from build123d import *

# Parameters (mm, degrees)
BOSS_EXTRUDE1_DEPTH = 600
FILLET1_R           = 5


with BuildPart() as part:
    # Sketch1 → Boss-Extrude1 (new body)
    with BuildSketch(Plane.XY):
        Polygon((-37.5, 50), (37.5, 50), (37.5, 40), (5, 34.269373127), (5, -34.269373127), (37.5, -40), (37.5, -50), (-37.5, -50), (-37.5, -40), (-5, -34.269373127), (-5, 34.269373127), (-37.5, 40), align=None)
    extrude(amount=BOSS_EXTRUDE1_DEPTH)

    # Fillet1
    fillet1_edges = [part.edges().sort_by_distance(p)[0] for p in [
        (5, 34.269373127, 300),
        (5, -34.269373127, 300),
        (37.5, -40, 300),
        (-37.5, -40, 300),
        (-5, -34.269373127, 300),
        (-5, 34.269373127, 300),
        (-37.5, 40, 300),
        (37.5, 40, 300),
    ]]
    fillet(fillet1_edges, radius=FILLET1_R)


solid = part.part
Input: part model. Units: mm. Frame: model coordinates. A direction names the side the tool comes from. Coordinates: 2 decimals unless noted, no trailing zeros. Order: outer loops, then holes, each group sorted by start corner. A loop starts at its lowest first (then second) coordinate and runs counter-clockwise, first axis right, second up. Notation, with made-up numbers: M 82.25,-5.75 L 138.25,-5.75 A21 ccw 138.25,3.25 Z; hole C 9.25,14.25 d10. An arc over 180 degrees is marked long. Write item = value, one per line. Start each with the question number.
(1) First-contact query: P1, Ø12, axis at y = -15, z = 436, coming from the +X side; P2, Ø2, axis at y = 12, z = 184.5, coming from the -X side; P3, Ø8, axis at x = 14, y = 36, coming from the -Z side. Flat tips, straight axial feed; report the tip coordinate or a pass-through.
(2) Line query: line 1 along X through (y, z) = (-5.5, 460); line 2 along Y through (x, z) = (-7.5, 305.5); line 3 along X through (y, z) = (-43.5, 83). Output: solid intervals per line, ascending. Write a range as [from, to].
(3) Section C-C on y = -8. Output: boundary loops of the cut face in (x, z), and give its area (3 significant figures).
(4) Pull-direction query (Y, two-part tool) for faces 4 (the flat face through (0, -3, 0)), 5 (the flat face through (-21.42, -37.165, 295.8)), 6 (the flat face through (-1, 50, 296)), 7 (the flat face through (-5, 0, 296)); classes: released by +Y, released by -Y, zero draft, split by the parting line, or undercut.
(5) Section B-B on z = 178. Output: boundary loops of the cut face in (x, y).
(6) Reachability of faces 1 (the flat face through (-21.08, 37.105, 295.8)), 2 (the flat face through (21.42, 37.165, 295.8)), 3 (the flat face through (0, -3, 600)) from +Z, -Z, +X, -X, +Y, -Y: full face, straight path, thin tool, end or side. Return the list, or none.
(7) Section A-A on x = -18. Output: boundary loops of the cut face in (y, z).
Result set:
q1.P1 = 5
q1.P2 = -5
q1.P3 = 0
q2.line_1 = [-5, 5]
q2.line_2 = [-50, -34.4], [34.4, 50]
q2.line_3 = [-37.45, 37.45]
q3.outline = M -5,0 L 5,0 L 5,600 L -5,600 Z
q3.area = 6,000 mm²
q4.face_4 = zero draft
q4.face_5 = undercut
q4.face_6 = released by +Y
q4.face_7 = undercut
q5.outline = M -37.5,-50 L 37.5,-50 L 37.5,-44.2 A5 ccw 33.37,-39.27 L 9.13,-35 A5 cw 5,-30.07 L 5,30.07 A5 cw 9.13,35 L 33.37,39.27 A5 ccw 37.5,44.2 L 37.5,50 L -37.5,50 L -37.5,44.2 A5 ccw -33.37,39.27 L -9.13,35 A5 cw -5,30.07 L -5,-30.07 A5 cw -9.13,-35 L -33.37,-39.27 A5 ccw -37.5,-44.2 Z
q6.face_1 = +Z, -Z, -X
q6.face_2 = +Z, -Z, +X
q6.face_3 = +Z, +X, -X, +Y, -Y
q7.outline = M -50,0 L -36.56,0 L -36.56,600 L -50,600 Z; M 36.56,0 L 50,0 L 50,600 L 36.56,600 Z
